Autodesk Fusion 360 part; units mm, degrees
sketch "草图1" plane through (0, 0, 0) normal (0, 0, 1) x (1, 0, 0)
  circle A0 centre (0, 0) radius 60
  circle A1 centre (-35, 45) radius 1.5
  circle A2 centre (-44.4343, 35.7155) radius 1.5
  circle A3 centre (-51.4731, 24.5055) radius 1.5
  circle A4 centre (-55.737, 11.9744) radius 1.5
  circle A5 centre (-56.9961, -1.2022) radius 1.5
  circle A6 centre (-55.1825, -14.314) radius 1.5
  circle A7 centre (-50.394, -26.6541) radius 1.5
  circle A8 centre (-42.8888, -37.5573) radius 1.5
  circle A9 centre (-33.0714, -46.4358) radius 1.5
  circle A10 centre (-21.4711, -52.8109) radius 1.5
  circle A11 centre (-8.7134, -56.339) radius 1.5
  circle A12 centre (4.5142, -56.8298) radius 1.5
  circle A13 centre (17.4983, -54.2569) radius 1.5
  circle A14 centre (29.5392, -48.759) radius 1.5
  circle A15 centre (39.9875, -40.6325) radius 1.5
  circle A16 centre (48.2801, -30.3155) radius 1.5
  circle A17 centre (53.97, -18.3641) radius 1.5
  circle A18 centre (56.7503, -5.4228) radius 1.5
  circle A19 centre (56.4711, 7.8109) radius 1.5
  circle A20 centre (53.1476, 20.6235) radius 1.5
  circle A21 centre (46.9589, 32.3243) radius 1.5
  circle A22 centre (38.2387, 42.2824) radius 1.5
  circle A23 centre (27.4569, 49.9612) radius 1.5
  circle A24 centre (15.195, 54.9464) radius 1.5
  circle A25 centre (2.1139, 56.9696) radius 1.5
  circle A26 centre (-11.0812, 55.9214) radius 1.5
  circle A27 centre (-23.6789, 51.8586) radius 1.5
  circle A28 centre (0, 0) radius 1.5
  dimension "d1" = 120
  dimension "d2" = 3
  dimension "d4" = 360
  dimension "d5" = 3
extrude "拉伸1" add sketch "草图1" along normal blind 3
Geometry check sheet. Reference: the model listing, model coordinates, mm. Round coordinates to 2 decimals unless told otherwise and drop trailing zeros. Write each loop counter-clockwise with the first axis right and the second up, starting at its lowest first coordinate (ties: lowest second). Pieces come first, ordered by that corner, then holes. Notation, with made-up numbers: (69, -7) - (88, -7) arc R28 cw to (88, 11) - close; hole circle Ø8 at (29, -3). An arc over 180 degrees is marked (long way). One line per item, written item: value.
1. Depth check by flat-ended pin: pin 1 Ø2.5 at (x, y) = (-11.08, 55.92) entering from -Z; pin 2 Ø1 at (x, z) = (-36, 0.5) entering from +Y. Enter the tip coordinate at first touch or a pass-through.
The answers:
pin 1: passes through
pin 2: stops at y = 48.37
2. Cross-section at B-B on x = -18. Record the boundary of the cut face in (y, z).
The answers:
outline: (-57.24, 0) - (57.24, 0) - (57.24, 3) - (-57.24, 3) - close
3. Mould release check, pull along Y, two halves, no side actions. Record for faces 1 (the face through (54.578, 20.173, 1.479)), 2 (the face through (30.231, -47.428, 1.479)): released by +Y, released by -Y, zero draft, split by the parting line, or undercut.
The answers:
face 1: undercut
face 2: undercut
4. Cross-section at C-C on y = -34. Record the boundary of the cut face in (x, z), and give its area (3 significant figures).
The answers:
outline: (-49.44, 0) - (49.44, 0) - (49.44, 3) - (-49.44, 3) - close
area: 297 mm^2
5. Scan lines: L1, parallel to X at y = -6, z = 0.4; L2, parallel to Y at x = 28, z = 2.25; L3, parallel to X at y = -52, z = 0.7. Record each from-to range of solid material in increasing order.
The answers:
L1: x = -59.7 to 55.37, 58.13 to 59.7
L2: y = -53.07 to 48.56, 51.36 to 53.07
L3: x = -29.93 to -22.73, -20.21 to 29.93
6. Cross-section at A-A on z = 1.3. Give the number of separate pieces and of enclosed holes in the cut face, and give its area (3 significant figures).
The answers:
separate pieces: 1
enclosed holes: 28
area: 11,100 mm^2
